```python
from build123d import *

# Parameters (mm, degrees)
F0_W     = 203.2
F0_H     = 127
F1_DEPTH = 127
F3_DEPTH = 76.2
F4_SIZE2 = 101.6
F4_SIZE  = 76.2
F5_R     = 5.08
F6_R     = 15.24
F7_DEPTH = 50.8
F8_R     = 19.05
F9_DEPTH = 127


with BuildPart() as f1:
    # F0 (on Front) → F1 (new body)
    with BuildSketch(Plane.XZ):
        Rectangle(F0_W, F0_H)
    extrude(amount=-F1_DEPTH)

    # F2 (on face) → F3 (cut)
    with BuildSketch(Plane.XZ):
        Polygon((-39.4764244556, 0), (-39.4764244556, -63.5), (101.6, -63.5), (101.6, 63.5), (0, 63.5), (0, 0), align=None)
    extrude(amount=-F3_DEPTH, mode=Mode.SUBTRACT)

    # F4
    f4_edges = [f1.edges().sort_by_distance(p)[0] for p in [
        (101.6, 101.6, 63.5),
    ]]
    f4_side = f1.faces().sort_by_distance((-21.771429, 74.385714, 63.5))[0]
    chamfer(f4_edges, length=F4_SIZE, length2=F4_SIZE2, reference=f4_side)

    # F5
    f5_edges = [f1.edges().sort_by_distance(p)[0] for p in [
        (101.6, 101.6, -63.5),
        (101.6, 101.6, -38.1),
        (25.4, 101.6, 63.5),
        (63.5, 76.2, 12.7),
        (63.5, 127, 12.7),
        (12.7, 76.2, 63.5),
        (0, 38.1, 63.5),
        (0, 38.1, 0),
        (101.6, 76.2, -50.8),
        (31.061788, 76.2, -63.5),
        (-39.476424, 76.2, -31.75),
        (0, 76.2, 31.75),
        (-19.738212, 76.2, 0),
        (-39.476424, 0, -31.75),
        (-19.738212, 0, 0),
        (-50.8, 0, 63.5),
        (0, 0, 31.75),
        (-101.6, 63.5, 63.5),
        (-38.1, 127, 63.5),
        (-70.538212, 0, -63.5),
        (-101.6, 0, 0),
        (-101.6, 63.5, -63.5),
        (-39.476424, 38.1, 0),
        (101.6, 127, -50.8),
        (0, 127, -63.5),
        (-39.476424, 38.1, -63.5),
        (-101.6, 127, 0),
    ]]
    fillet(f5_edges, radius=F5_R)

    # F6 (on face) → F7 (cut, through all)
    with BuildSketch(Plane.XZ.offset(-76.2)):
        with Locations((16.4035755444, -17.78)):
            Circle(F6_R)
    extrude(amount=-F7_DEPTH, mode=Mode.SUBTRACT)

    # F8 (on face) → F9 (cut, through all)
    with BuildSketch(Plane.XY.offset(63.5)):
        with Locations((-60.96, 88.9)):
            Circle(F8_R)
    extrude(amount=-F9_DEPTH, mode=Mode.SUBTRACT)


solid = f1.part
```
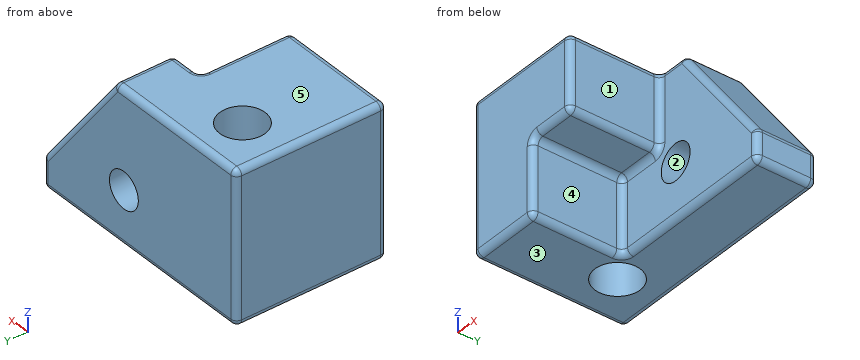
Input: part model. Units: mm. Frame: model coordinates. Face numbers are marked on the shaded views. A direction names the side the tool comes from. Coordinates: 2 decimals unless noted, no trailing zeros. Loops run counter-clockwise (first coordinate to the right, second up) from the corner with the lowest first, then second, coordinate; pieces in that order, holes last. Notation, with made-up numbers: (4.25, 37) - (53.25, 37) arc R8 cw to (53.25, 47) - close; hole circle Ø6 at (-16.5, 77). An arc over 180 degrees is marked (long way). Answer in a Markdown table with one row per item.
(1) Set-up query: the marked faces 4 and 5. Return all of +Z, -Z, +X, -X, +Y, -Y with unobstructed straight access to the full face (end or side cutting, diameter ignored); none if empty.
Model answer:
| item | result |
|---|---|
| face 4 | -Z, +X, -Y |
| face 5 | +Z, +X, -X, +Y, -Y |
(2) Material intervals for L1, parallel to Y at x = -60.96, z = 13; L2, parallel to X at y = 101, z = -17 (3 decimals); L3, parallel to X at y = 102, z = -17 (3 decimals), sorted ascending. Write a range as from..to.
Model answer:
| item | result |
|---|---|
| L1 | y = 0..69.85, 107.95..127 |
| L2 | x = -101.6..-75.674, -46.246..1.184, 31.624..85.775 |
| L3 | x = -101.6..-74.791, -47.129..1.184, 31.624..85.775 |
(3) Cut plane C-C on z = -17.78. Count the separate pieces of the cut face and the enclosed holes in it, plus the area to 3 significant figures.
Model answer:
| item | result |
|---|---|
| separate pieces | 2 |
| enclosed holes | 1 |
| area | 11,600 mm² |
(4) Cut plane A-A on x = -60.96. Output: boundary loops of the cut face in (y, z), plus the area to 3 significant figures.
Model answer:
| item | result |
|---|---|
| outline | (0, -58.42) arc R5.08 ccw to (5.08, -63.5) - (69.85, -63.5) - (69.85, 63.5) - (5.08, 63.5) arc R5.08 ccw to (0, 58.42) - close; (107.95, -63.5) - (121.92, -63.5) arc R5.08 ccw to (127, -58.42) - (127, 58.42) arc R5.08 ccw to (121.92, 63.5) - (107.95, 63.5) - close |
| area | 11,300 mm² |
(5) Cut plane D-D on y = 117. Output: boundary loops of the cut face in (x, z).
Model answer:
| item | result |
|---|---|
| outline | (-101.6, -58.42) arc R5.08 ccw to (-96.52, -63.5) - (96.52, -63.5) arc R5.08 ccw to (101.6, -58.42) - (101.6, -39.79) arc R5.08 ccw to (100.58, -36.75) - (26.92, 61.47) arc R5.08 ccw to (22.86, 63.5) - (-96.52, 63.5) arc R5.08 ccw to (-101.6, 58.42) - close; hole circle Ø30.48 at (16.4, -17.78) |
(6) Pin query (flat end, axial travel): P1, Ø2, axis at x = 71, z = -37, coming from the -Y side; P2, Ø5, axis at y = 79, z = 30, coming from the +X side. Return the tip coordinate at first contact, or that it passes through.
Model answer:
| item | result |
|---|---|
| P1 | stops at y = 76.2 |
| P2 | stops at x = 52.04 |
(7) Mould query, pull axis Z, two halves, no side actions, for the marked faces 1, 2 and 3. Classes: pulls with the +Z half, pulls with the -Z half, needs draft (parallel to the pull), parting line crosses it, or undercut.
Model answer:
| item | result |
|---|---|
| face 1 | needs draft |
| face 2 | undercut |
| face 3 | pulls with the -Z half |
(8) Cut plane B-B on y = 88.9. Output: boundary loops of the cut face in (x, z), plus the area to 3 significant figures.
Model answer:
| item | result |
|---|---|
| outline | (-101.6, -58.42) arc R5.08 ccw to (-96.52, -63.5) - (-80.01, -63.5) - (-80.01, 63.5) - (-96.52, 63.5) arc R5.08 ccw to (-101.6, 58.42) - close; (-41.91, -63.5) - (96.52, -63.5) arc R5.08 ccw to (101.6, -58.42) - (101.6, -39.79) arc R5.08 ccw to (100.58, -36.75) - (26.92, 61.47) arc R5.08 ccw to (22.86, 63.5) - (-41.91, 63.5) - close; hole circle Ø30.48 at (16.4, -17.78) |
| area | 16,300 mm² |
